from build123d import *

# Parameters (mm, degrees)
F0_R     = 40
F0_R_2   = 2.5
F1_DEPTH = 2.5


with BuildPart() as f1:
    # F0 (on Front) → F1 (new body, symmetric)
    with BuildSketch(Plane.XZ):
        Circle(F0_R)
        with BuildLine():
            ThreePointArc((-5, -30.594117), (-21.92031, -21.92031), (-30.594117, -5))
            Line((-30.594117, -5), (-5.59017, -5))
            ThreePointArc((-5.59017, -5), (-5.303301, -5.303301), (-5, -5.59017))
            Line((-5, -5.59017), (-5, -30.594117))
        make_face(mode=Mode.SUBTRACT)
        with BuildLine():
            Line((5, -30.594117), (5, -5.59017))
            ThreePointArc((5, -5.59017), (5.303301, -5.303301), (5.59017, -5))
            Line((5.59017, -5), (30.594117, -5))
            ThreePointArc((30.594117, -5), (21.92031, -21.92031), (5, -30.594117))
        make_face(mode=Mode.SUBTRACT)
        with BuildLine():
            Line((-5, 30.594117), (-5, 5.59017))
            ThreePointArc((-5, 5.59017), (-5.303301, 5.303301), (-5.59017, 5))
            Line((-5.59017, 5), (-30.594117, 5))
            ThreePointArc((-30.594117, 5), (-21.92031, 21.92031), (-5, 30.594117))
        make_face(mode=Mode.SUBTRACT)
        Circle(F0_R_2, mode=Mode.SUBTRACT)
        with BuildLine():
            ThreePointArc((5.59017, 5), (5.303301, 5.303301), (5, 5.59017))
            Line((5, 5.59017), (5, 30.594117))
            ThreePointArc((5, 30.594117), (21.92031, 21.92031), (30.594117, 5))
            Line((30.594117, 5), (5.59017, 5))
        make_face(mode=Mode.SUBTRACT)
    extrude(amount=F1_DEPTH, both=True)


solid = f1.part
Design review of the part built by this model. Coordinates are the model's own, in mm. A direction names the side the tool comes from. Round coordinates to 2 decimals unless told otherwise and drop trailing zeros. Write each loop counter-clockwise with the first axis right and the second up, starting at its lowest first coordinate (ties: lowest second). Pieces come first, ordered by that corner, then holes.
Item 1: Consider section B-B on y = 1.3. Give the boundary of the cut face in (x, z), and give its area (3 significant figures).
Item 2: For faces 4 (the flat face through (-1, 2.5, -8)), 5 (the flat face through (-18, 0, -5)), list the 3-axis set-ups (+Z, -Z, +X, -X, +Y, -Y) from which the entire face can be reached by the end or side of a thin tool; tool diameter is ignored.
Item 3: Consider section C-C on x = 0. Give the boundary of the cut face in (y, z), and give its area (3 significant figures).
Item 4: Consider section D-D on z = 21. Give the boundary of the cut face in (x, y), and give its area (3 significant figures).
Item 5: Consider section A-A on z = 0. Give the boundary of the cut face in (x, y), and give its area (3 significant figures).
Item 6: Draft analysis for pull direction X (two halves, no side actions). For faces 1 (the cylindrical face through (-8.67, -0.04, -39.05)), 2 (the flat face through (-1, -2.5, -8)), 3 (the flat face through (-5, 0, 18)), state which applies: released by +X, released by -X, zero draft, split by the parting line, or undercut.
Item 7: Wall thickness on L1, parallel to Z at x = 0, y = -0.2; L2, parallel to X at y = -0.9, z = -6; L3, parallel to Z at x = 18, y = -0.75: over which ranges is each line inside the solid? List them lowest first.
Item 8: For pin 1 Ø1.5 at (y, z) = (1, -19.5) entering from +X; pin 2 Ø1.5 at (y, z) = (0, -31.5) entering from -X; pin 3 Ø1.5 at (x, y) = (20, -0.5) entering from -Z, all flat-tipped, find the tip position at first contact; note any pin that passes through.
Check values:
1. outline: circle Ø80 at (0, 0); hole (-30.59, -5) arc R31 ccw to (-5, -30.59) - (-5, -5.59) arc R7.5 cw to (-5.59, -5) - close; hole (-30.59, 5) - (-5.59, 5) arc R7.5 cw to (-5, 5.59) - (-5, 30.59) arc R31 ccw to start; hole circle Ø5 at (0, 0); hole (5, -30.59) arc R31 ccw to (30.59, -5) - (5.59, -5) arc R7.5 cw to (5, -5.59) - close; hole (5, 5.59) arc R7.5 cw to (5.59, 5) - (30.59, 5) arc R31 ccw to (5, 30.59) - close
1. area: 3,120 mm2
2. face 4: +Z, -Z, +X, -X, +Y
2. face 5: +Y, -Y
3. outline: (-2.5, -40) - (2.5, -40) - (2.5, -2.5) - (-2.5, -2.5) - close; (-2.5, 2.5) - (2.5, 2.5) - (2.5, 40) - (-2.5, 40) - close
3. area: 375 mm2
4. outline: (-34.04, -2.5) - (-22.8, -2.5) - (-22.8, 2.5) - (-34.04, 2.5) - close; (-5, -2.5) - (5, -2.5) - (5, 2.5) - (-5, 2.5) - close; (22.8, -2.5) - (34.04, -2.5) - (34.04, 2.5) - (22.8, 2.5) - close
4. area: 162 mm2
5. outline: (-40, -2.5) - (-2.5, -2.5) - (-2.5, 2.5) - (-40, 2.5) - close; (2.5, -2.5) - (40, -2.5) - (40, 2.5) - (2.5, 2.5) - close
5. area: 375 mm2
6. face 1: split by the parting line
6. face 2: zero draft
6. face 3: undercut
7. L1: z = -40 to -2.5, 2.5 to 40
7. L2: x = -39.55 to -30.41, -5 to 5, 30.41 to 39.55
7. L3: z = -35.72 to -25.24, -5 to 5, 25.24 to 35.72
8. pin 1: stops at x = 35.33
8. pin 2: stops at x = -25.58
8. pin 3: stops at z = -35.06
